Print and shaded views of the part. All mm, measured from the part's lowest x, y and z. Give positions to 0.01 mm unless a question says otherwise; leave off trailing zeros. Loops run counter-clockwise (first coordinate to the right, second up) from the corner with the lowest first, then second, coordinate; pieces in that order, holes last. Notation, with made-up numbers: (13.5, 70.25) -> (50.5, 70.25) arc R17 ccw to (50.5, 90.25) -> close; hole circle Ø10 at (74.5, 83). An arc over 180 degrees is marked (long way). Write each question's results on one line, items separated by ' | '. Start each with the question number.
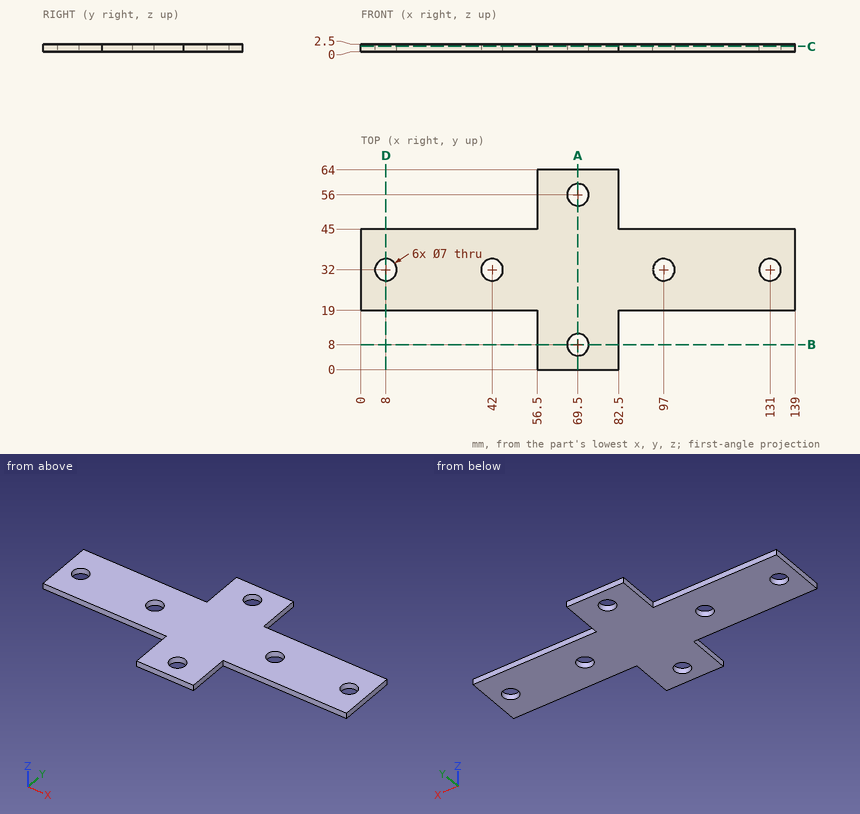
Q1. Saw through at A-A, the plane x = 69.5. List the corners of the cut face in (y, z).
Q2. Saw through at D-D, the plane x = 8. List the corners of the cut face in (y, z), then the cut area to 3 significant figures.
Q3. Wall check: L1, parallel to Y at x = 69.5, z = 1.65; L2, parallel to X at y = 30.5, z = 1.1; L3, parallel to Y at x = 97, z = 0.9. Give the ranges that are in metal, low to high.
Q4. Drop flat-ended pins along their axis: pin 1 (0.8 mm diameter, centred on x = 32.5, z = 1.5, fed in from -Y); pin 2 (1.2 mm diameter, centred on y = 52, z = 1.5, fed in from -X); pin 3 (0.8 mm diameter, centred on x = 100.5, z = 1.5, fed in from +Y). Give the stop position or say it passes through.
Q5. Saw through at C-C, the plane z = 1.7. List the corners of the cut face in (x, y), then the cut area to 3 significant figures.
Q6. Saw through at B-B, the plane y = 8. List the corners of the cut face in (x, z), then the cut area to 3 significant figures.
Answer block:
1) outline: (0, 0) -> (4.5, 0) -> (4.5, 2.5) -> (0, 2.5) -> close; (11.5, 0) -> (52.5, 0) -> (52.5, 2.5) -> (11.5, 2.5) -> close; (59.5, 0) -> (64, 0) -> (64, 2.5) -> (59.5, 2.5) -> close
2) outline: (19, 0) -> (28.5, 0) -> (28.5, 2.5) -> (19, 2.5) -> close; (35.5, 0) -> (45, 0) -> (45, 2.5) -> (35.5, 2.5) -> close | area: 47.5 mm2
3) L1: y = 0 to 4.5, 11.5 to 52.5, 59.5 to 64 | L2: x = 0 to 4.84, 11.16 to 38.84, 45.16 to 93.84, 100.16 to 127.84, 134.16 to 139 | L3: y = 19 to 28.5, 35.5 to 45
4) pin 1: stops at y = 19 | pin 2: stops at x = 56.5 | pin 3: stops at y = 45
5) outline: (0, 19) -> (56.5, 19) -> (56.5, 0) -> (82.5, 0) -> (82.5, 19) -> (139, 19) -> (139, 45) -> (82.5, 45) -> (82.5, 64) -> (56.5, 64) -> (56.5, 45) -> (0, 45) -> close; hole circle Ø7 at (8, 32); hole circle Ø7 at (42, 32); hole circle Ø7 at (69.5, 8); hole circle Ø7 at (69.5, 56); hole circle Ø7 at (97, 32); hole circle Ø7 at (131, 32) | area: 4,370 mm2
6) outline: (56.5, 0) -> (66, 0) -> (66, 2.5) -> (56.5, 2.5) -> close; (73, 0) -> (82.5, 0) -> (82.5, 2.5) -> (73, 2.5) -> close | area: 47.5 mm2
